Autodesk Inventor part; units mm, degrees
ref_plane "Work Plane1" through (6, 0, 0) normal (1, 0, 0) x (0, 0, -1)
ref_plane "YZ Plane" through (0, 0, 0) normal (1, 0, 0) x (0, 1, 0)
ref_plane "XZ Plane" through (0, 0, 0) normal (0, 1, 0) x (-1, 0, 0)
sketch "Sketch2" plane through (0, 0, 0) normal (1, 0, 0) x (0, 1, 0)
  line L0 (0, 0) -> (15, 0)
  line L1 (15, 0) -> (15, -10)
  line L2 (15, -10) -> (0, -10)
  line L3 (0, -10) -> (0, 0)
  dimension "d4" = 15
  dimension "d5" = 10
extrude "Extrusion2" add sketch "Sketch2" along normal blind 12
sketch "Sketch3" plane through (0, 0, 0) normal (0, 0, 1) x (1, 0, 0)
  line L0 (0, 0) -> (1, 0)
  line L1 (0, 0) -> (12, 0)
  line L2 (1, 0) -> (1, 13.5)
  line L3 (1, 13.5) -> (11, 13.5)
  line L4 (11, 13.5) -> (11, 0)
  line L5 (11, 0) -> (1, 0)
  dimension "d8" = 1
  dimension "d9" = 13.5
  dimension "d10" = 10
extrude "Extrusion3" cut sketch "Sketch3" against normal blind 8
sketch "Sketch4" plane through (0, 0, -10) normal (0, 0, -1) x (-1, 0, 0)
  line L0 (0, 15) -> (-12, 15)
  line L1 (0, 0) -> (-12, 0)
  line L2 (-12, 15) -> (0, 15)
  line L3 (0, 15) -> (0, 0)
  line L4 (0, 0) -> (-12, 0)
  line L5 (-12, 0) -> (-12, 15)
extrude "Extrusion4" add sketch "Sketch4" along normal blind 2
sketch "Sketch5" plane through (0, 0, -8) normal (0, 0, 1) x (1, 0, 0)
  line L0 (1, 13.5) -> (11, 13.5)
  line L1 (6, 13.5) -> (6, 10)
  line L2 (6, 10) -> (6, 3.5)
  circle A0 centre (6, 10) radius 1.2295
  circle A1 centre (6, 3.5) radius 1.2295
  point P0 (0, 0)
  dimension "d15" = 3.5
  dimension "d16" = 6.5
  dimension "d17" = 2.459
  dimension "d18" = 2.459
extrude "Extrusion5" cut sketch "Sketch5" against normal blind 4
sketch "Sketch6" plane through (0, 0, -8) normal (0, 0, 1) x (1, 0, 0)
  circle A0 centre (6, 10) radius 1.2295
  circle A1 centre (6, 10) radius 2.7
  circle A2 centre (6, 3.5) radius 1.2295
  circle A3 centre (6, 3.5) radius 2.7
  point P0 (0, 0)
  dimension "d21" = 5.4
  dimension "d22" = 5.4
extrude "Extrusion6" cut sketch "Sketch6" against normal blind 1.1
sketch "Sketch15" plane through (12, 0, 0) normal (1, 0, 0) x (0, 0, -1)
  line L0 (0, 15) -> (12, 15)
  line L1 (12, 15) -> (12, 0)
  line L2 (0, 15) -> (12, 15)
  line L3 (12, 15) -> (12, 0)
  line L4 (12, 0) -> (0, 0)
  line L5 (0, 0) -> (0, 15)
extrude "Extrusion14" add sketch "Sketch15" along normal blind 4
ref_plane "Work Plane1" through (6, 0, 0) normal (1, 0, 0) x (0, 0, -1)
mirror "Mirror1" about plane through (6, 0, 0) normal (1, 0, 0) of "Extrusion14"
sketch "Sketch16" plane through (1, 0, -8) normal (0, -1, 0) x (1, 0, 0)
  line L0 (10, 0) -> (0, 0)
  line L1 (5, 0) -> (7.5, 0)
  line L2 (7.5, 0) -> (7.5, -4)
  line L3 (-5, -4) -> (15, -4)
  line L4 (7.5, -4) -> (2.5, -4)
  line L5 (2.5, -4) -> (2.5, 0)
  line L6 (2.5, 0) -> (5, 0)
  point P0 (-1, 8)
  dimension "d61" = 2.5
  dimension "d62" = 4
  dimension "d63" = 5
  dimension "d64" = 4
extrude "Extrusion15" add sketch "Sketch16" along normal blind 10
sketch "Sketch18" plane through (0, 0, -12) normal (0, 0, -1) x (-1, 0, 0)
  line L0 (-16, 15) -> (4, 15)
  line L1 (4, 0) -> (-3.5, 0)
  line L2 (-16, 15) -> (4, 15)
  line L3 (4, 15) -> (4, 0)
  line L4 (4, 0) -> (-16, 0)
  line L5 (-16, 0) -> (-16, 15)
  line L6 (-8.5, -10) -> (-3.5, -10)
  line L7 (-3.5, 0) -> (-8.5, 0)
  line L8 (-8.5, 0) -> (-8.5, -10)
  line L9 (-8.5, -10) -> (-3.5, -10)
  line L10 (-3.5, -10) -> (-3.5, 0)
  circle A0 centre (-6, 3.5) radius 1.2295
  circle A1 centre (-6, 3.5) radius 1.2295
  circle A2 centre (-6, 10) radius 1.2295
  circle A3 centre (-6, 10) radius 1.2295
  point P0 (0, 0)
extrude "Extrusion16" add sketch "Sketch18" along normal blind 1
sketch "Sketch19" plane through (16, 0, 0) normal (1, 0, 0) x (0, 0, -1)
  line L0 (0, 15) -> (13, 15)
  line L1 (0, 15) -> (0, 40)
  line L2 (13, 45) -> (13, 15)
  line L3 (13, 56) -> (13, 45)
  line L4 (0, 45) -> (0, 40)
  line L5 (0, 45) -> (-5, 45)
  line L6 (13, 60) -> (13, 56)
  line L7 (-5, 77) -> (0, 77)
  line L8 (0, 77) -> (13, 61)
  line L9 (13, 61) -> (13, 60)
  line L10 (0, 61) -> (-5, 77)
  line L11 (0, 61) -> (-5, 45)
  point P0 (0, 0)
extrude "Extrusion17" add sketch "Sketch19" against normal blind 20
properties part number "30mm_x_20mm"
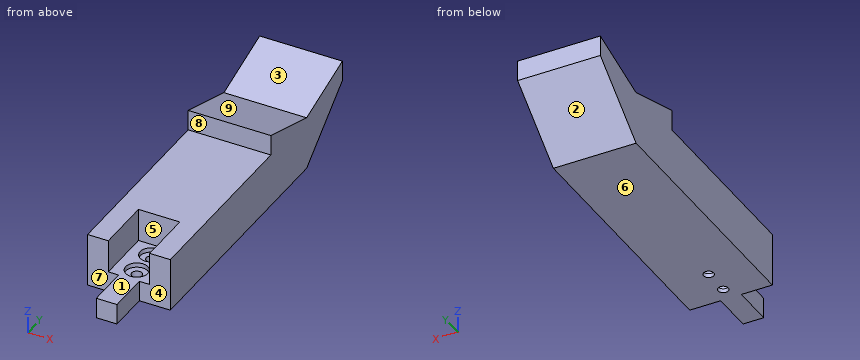
Part model, mm, in its own coordinate system. Face numbers are marked on the shaded views. A direction names the side the tool comes from. Give positions to 0.01 mm unless a question says otherwise; leave off trailing zeros. Loops run counter-clockwise (first coordinate to the right, second up) from the corner with the lowest first, then second, coordinate; pieces in that order, holes last. Notation, with made-up numbers: M 55.5,46.5 L 102.5,46.5 A11 ccw 102.5,54.5 Z; hole C 75.5,72 d5. An arc over 180 degrees is marked long. Put each result on its own line as item: value. Start each with the question number.
1) Saw through at B-B (z = 3.25). List the corners of the cut face in (x, y).
2) Saw through at D-D (x = 13.25). List the corners of the cut face in (y, z).
3) Flat gauge pins, fed straight in: pin 1 (4 mm diameter, centred on y = -6.5, z = -9.5, fed in from +X); pin 2 (6 mm diameter, centred on x = 0, z = -11, fed in from -Y); pin 3 (8 mm diameter, centred on x = 5.5, z = -10.5, fed in from +Y). Where does each tip first touch, or does it go through?
4) Saw through at A-A (y = 10). List the corners of the cut face in (x, z), then the cut area to 3 significant figures.
5) 3-axis set-ups, long thin cutter, end or side, ignore diameter. For the marked faces 5, 6, 7, 8 and 9: which of +Z, -Z, +X, -X, +Y, -Y reach the whole face in a straight line?
6) Pull direction Y, two halves, no side cores. Call the marked faces 1, 2, 3 and 4: +Y half, -Y half, draft (parallel to the pull), parting line (faces both ways), or undercut.
7) Probe probe 1 along Y at (x, z) = (6, -12.4); probe 2 along Y at (x, z) = (6, -8.8); probe 3 along X at (y, z) = (10, -12.55). List the from-to ranges inside material, lowest first.
8) Saw through at C-C (x = 6). List the corners of the cut face in (y, z), then the cut area to 3 significant figures.
Numbers:
1. outline: M -4,45 L 16,45 L 16,50.6 L -4,50.6 Z; M -4,71.4 L 16,71.4 L 16,77 L -4,77 Z
2. outline: M 0,-13 L 61,-13 L 77,0 L 77,5 L 61,0 L 45,5 L 45,0 L 0,0 Z
3. pin 1: x = 8.5
3. pin 2: y = 0
3. pin 3: y = 69
4. outline: M -4,-13 L 4.77,-13 L 4.77,-9.1 L 3.3,-9.1 L 3.3,-8 L 1,-8 L 1,0 L -4,0 Z; M 7.23,-13 L 16,-13 L 16,0 L 11,0 L 11,-8 L 8.7,-8 L 8.7,-9.1 L 7.23,-9.1 Z
4. area: 164 mm^2
5. face 5: +Z, -Y
5. face 6: -Z, +X, -X, +Y, -Y
5. face 7: +Z, -Z, -X, -Y
5. face 8: +Z, +X, -X, -Y
5. face 9: +Z, +X, -X
6. face 1: draft
6. face 2: +Y half
6. face 3: undercut
6. face 4: -Y half
7. probe 1: -10 to 2.27, 4.73 to 8.77, 11.23 to 61.74
7. probe 2: -10 to 0.8, 6.2 to 7.3, 12.7 to 66.17
7. probe 3: -4 to 4.77, 7.23 to 16
8. outline: M -10,-13 L 2.27,-13 L 2.27,-9.1 L 0.8,-9.1 L 0.8,-8 L -10,-8 Z; M 4.73,-13 L 8.77,-13 L 8.77,-9.1 L 7.3,-9.1 L 7.3,-8 L 6.2,-8 L 6.2,-9.1 L 4.73,-9.1 Z; M 11.23,-13 L 61,-13 L 77,0 L 77,5 L 61,0 L 45,5 L 45,0 L 13.5,0 L 13.5,-8 L 12.7,-8 L 12.7,-9.1 L 11.23,-9.1 Z
8. area: 888 mm^2
